from build123d import *

# Parameters (mm, degrees)
SKETCH_1_R          = 2.75
EXTRUDE_1_DEPTH     = 1
SKETCH_2_W          = 5
SKETCH_2_H          = 3.5
SKETCH_2_W_2        = 2
SKETCH_2_H_2        = 6.5
CUT_EXTRUDE_1_DEPTH = 2
SKETCH_3_W          = 14.891608376
SKETCH_3_H          = 2
EXTRUDE_2_DEPTH     = 5
FILLET_1_R          = 2


with BuildPart() as part:
    # 草图1 → 凸台-拉伸1 (new body)
    with BuildSketch(Plane.XY):
        with BuildLine():
            Line((-7.445804188, 14.5), (7.445804188, 14.5))
            ThreePointArc((7.445804188, 14.5), (0, -16.3), (-7.445804188, 14.5))
        make_face()
        Circle(SKETCH_1_R, mode=Mode.SUBTRACT)
    extrude(amount=EXTRUDE_1_DEPTH)

    # 草图2 → 切除-拉伸1 (cut, through all)
    with BuildSketch(Plane.XY.offset(1)):
        with Locations((-16.3, 0)):
            Rectangle(SKETCH_2_W, SKETCH_2_H)
        with Locations((16.2, 0)):
            Rectangle(SKETCH_2_W_2, SKETCH_2_H_2)
    extrude(amount=-CUT_EXTRUDE_1_DEPTH, mode=Mode.SUBTRACT)

    # 草图3 → 凸台-拉伸2 (add)
    with BuildSketch(Plane.XY.offset(1)):
        with Locations((0, 13.5)):
            Rectangle(SKETCH_3_W, SKETCH_3_H)
    extrude(amount=EXTRUDE_2_DEPTH)

    # 圆角1
    fillet_1_edges = [part.edges().sort_by_distance(p)[0] for p in [
        (0, 12.5, 1),
    ]]
    fillet(fillet_1_edges, radius=FILLET_1_R)


solid = part.part
The model under review builds one solid part; all positions refer to its coordinate system, in mm. A direction names the side the tool comes from. Coordinates: 2 decimals unless noted, no trailing zeros. Loops run counter-clockwise (first coordinate to the right, second up) from the corner with the lowest first, then second, coordinate; pieces in that order, holes last.
(1) Consider section D-D, the plane x = -7. Give the boundary of the cut face in (y, z).
Determined:
outline: (-14.72, 0) - (14.5, 0) - (14.5, 6) - (12.5, 6) - (12.5, 3) arc R2 cw to (10.5, 1) - (-14.72, 1) - close
(2) Wall thickness on L1, parallel to Y at x = 0, z = 0.55; L2, parallel to Z at x = -8.5, y = 12.5; L3, parallel to Y at x = -7, z = 5.3: over which ranges is each line inside the solid? List them lowest first.
Determined:
L1: y = -16.3 to -2.75, 2.75 to 14.5
L2: z = 0 to 1
L3: y = 12.5 to 14.5
(3) Consider section C-C, the plane z = 4.15. Give the boundary of the cut face in (x, y).
Determined:
outline: (-7.45, 12.5) - (7.45, 12.5) - (7.45, 14.5) - (-7.45, 14.5) - close
(4) Draft analysis for pull direction X (two halves, no side actions). For faces 4 (the flat face through (0, 12.5, 4)), 5 (the cylindrical face through (-0.436, -16.294, 0.493)), 6 (the flat face through (-13.8, 0, 0.5)), 7 (the cylindrical face through (-0.596, -2.685, 0.493)), state which applies: +X half, -X half, draft (parallel to the pull), parting line (faces both ways), or undercut.
Determined:
face 4: draft
face 5: parting line
face 6: -X half
face 7: undercut
(5) Insertion check: P1, Ø0.8, axis at x = -15, z = 0.5, coming from the -Y side; P2, Ø3, axis at x = 10, y = 2.5, coming from the +Z side; P3, Ø2, axis at y = 4.5, z = 2.5, coming from the +X side; P4, Ø8, axis at x = -5.5, y = 7, coming from the +Z side. Each pin has a flat end and moves straight along its axis. Give the tip position at first contact, or say it passes through.
Determined:
P1: stops at y = -7.25
P2: stops at z = 1
P3: passes through
P4: stops at z = 1.06
(6) Tool access review of faces 1 (the flat face through (-7.446, 13, 3)), 2 (the flat face through (-15, 1.75, 0.5)), 3 (the flat face through (15.2, 0, 0.5)): name each direction out of +Z, -Z, +X, -X, +Y, -Y from which nothing blocks a thin tool from reaching the whole face with its end or side.
Determined:
face 1: +Z, -X, +Y, -Y
face 2: +Z, -Z, -X
face 3: +Z, -Z, +X
(7) Consider section A-A, the plane y = 0. Give the boundary of the cut face in (x, z), plus the area to 3 significant figures.
Determined:
outline: (-13.8, 0) - (-2.75, 0) - (-2.75, 1) - (-13.8, 1) - close; (2.75, 0) - (15.2, 0) - (15.2, 1) - (2.75, 1) - close
area: 23.5 mm2
(8) Consider section B-B, the plane x = 0. Give the boundary of the cut face in (y, z).
Determined:
outline: (-16.3, 0) - (-2.75, 0) - (-2.75, 1) - (-16.3, 1) - close; (2.75, 0) - (14.5, 0) - (14.5, 6) - (12.5, 6) - (12.5, 3) arc R2 cw to (10.5, 1) - (2.75, 1) - close
